```python
from build123d import *

# Parameters (mm, degrees)
F0_W     = 32
F0_H     = 32
F1_DEPTH = 1.6
F2_W     = 5.95
F2_H     = 3.7
F3_DEPTH = 4.75
F4_W     = 16.95
F4_H     = 16.95
F5_DEPTH = 7.75
F6_R     = 7.575
F7_DEPTH = 15.5
F8_R     = 1
F9_DEPTH = 7.75


# Not quite as in the source:
# - a pattern or mirror of a feature is missing from the dataset's text; its kind, count and spacing are read off the source's solid


with BuildPart() as f1:
    # F0 (on Front) → F1 (new body)
    with BuildSketch(Plane.XZ):
        Rectangle(F0_W, F0_H)
    extrude(amount=F1_DEPTH)

    # F2 (on face) → F3 (join)
    with BuildSketch(Plane.XZ.offset(1.6)):
        with Locations((-7.275, -14.15)):
            Rectangle(F2_W, F2_H)
    extrude(amount=F3_DEPTH)

    # F4 (on face) → F5 (join)
    with BuildSketch(Plane(origin=(0, 0, 0), x_dir=(-1, 0, 0), z_dir=(0, 1, 0))):
        Rectangle(F4_W, F4_H)
    extrude(amount=F5_DEPTH)

    # F6 (on face) → F7 (join)
    with BuildSketch(Plane(origin=(0, 7.75, 0), x_dir=(-1, 0, 0), z_dir=(0, 1, 0))):
        Circle(F6_R)
    extrude(amount=F7_DEPTH)

    # F8 (on face) → F9 (join)
    with BuildSketch(Plane(origin=(0, 0, 0), x_dir=(-1, 0, 0), z_dir=(0, 1, 0))):
        with BuildLine():
            Line((-8.475, 2.4), (-10, 2.4))
            ThreePointArc((-10, 2.4), (-12.4, 0), (-10, -2.4))
            Line((-10, -2.4), (-8.475, -2.4))
            Line((-8.475, -2.4), (-8.475, 2.4))
        make_face()
        with Locations((-10, 0)):
            Circle(F8_R, mode=Mode.SUBTRACT)
    f9 = extrude(amount=F9_DEPTH)

    # F9_copies: F9 across plane
    add(f9.mirror(Plane(origin=(0, 0, 0), x_dir=(0, 0, -1), z_dir=(-1, 0, 0))))


solid = f1.part
```
Read the model definition and answer for the solid it produces. Units are mm, in the model's axes. A direction names the side the tool comes from. Give positions to 0.01 mm unless a question says otherwise; leave off trailing zeros. Loops run counter-clockwise (first coordinate to the right, second up) from the corner with the lowest first, then second, coordinate; pieces in that order, holes last.
Item 1: The mould has two halves that part along Z. Classify faces 1 (the flat face through (-10, 0, 0)), 2 (the cylindrical face through (-10.8, 3.8, -0.6)), 3 (the flat face through (9, 4, 2.4)), 4 (the flat face through (9, 4, -2.4)): released by +Z, released by -Z, zero draft, split by the parting line, or undercut.
Item 2: Each of these flat-tipped pins is pushed along its axis until it touches: pin 1 Ø2.5 at (x, z) = (-10, 0) entering from -Y; pin 2 Ø0.6 at (x, z) = (-10, -0.5) entering from +Y; pin 3 Ø5 at (x, y) = (-9.5, 14.5) entering from -Z. Where does it stop, or does it pass through?
Item 3: For faces 5 (the flat face through (0, 7.75, 8)), 6 (the flat face through (-10.25, -4, -14)), 7 (the flat face through (0, 4, -8.475)), 8 (the cylindrical face through (-12.4, 3.82, 0.05)), determine the directions among +Z, -Z, +X, -X, +Y, -Y from which every point of the face is accessible in a straight line to the end or side of a thin tool.
Item 4: The part is cut by section C-C (x = 0). Write down the section's boundary in (y, z) (3 decimals), and give its area (3 significant figures).
Item 5: The part is cut by section A-A (y = 0.5). Write down the section's boundary in (x, z) (3 decimals).
Item 6: Find the intervals of material crossed by line 1 along Z through (x, y) = (-10, 6); line 2 along Y through (x, z) = (3, 12); line 3 along Y through (x, z) = (1, -7), in increasing order.
Item 7: The part is cut by section B-B (z = 0). Write down the section's boundary in (x, y) (3 decimals).
Item 8: The part is cut by section D-D (y = 16.5). Write down the section's boundary in (x, z) (3 decimals).
Taken from the geometry:
1. face 1: undercut
1. face 2: undercut
1. face 3: released by +Z
1. face 4: released by -Z
2. pin 1: stops at y = -1.6
2. pin 2: stops at y = 0
2. pin 3: stops at z = -2.89
3. face 5: +Y
3. face 6: +Z, -Z, -X, -Y
3. face 7: -Z, +X, -X, +Y
3. face 8: -X, +Y
4. outline: (-1.6, -16) - (0, -16) - (0, -8.475) - (7.75, -8.475) - (7.75, -7.575) - (23.25, -7.575) - (23.25, 7.575) - (7.75, 7.575) - (7.75, 8.475) - (0, 8.475) - (0, 16) - (-1.6, 16) - close
4. area: 417 mm2
5. outline: (-10, -2.4) - (-8.475, -2.4) - (-8.475, -8.475) - (8.475, -8.475) - (8.475, -2.4) - (10, -2.4) arc R2.4 ccw to (10, 2.4) - (8.475, 2.4) - (8.475, 8.475) - (-8.475, 8.475) - (-8.475, 2.4) - (-10, 2.4) arc R2.4 ccw to start; hole circle Ø2 at (-10, 0); hole circle Ø2 at (10, 0)
6. line 1: z = -2.4 to -1, 1 to 2.4
6. line 2: y = -1.6 to 0
6. line 3: y = -1.6 to 23.25
7. outline: (-16, -1.6) - (16, -1.6) - (16, 0) - (12.4, 0) - (12.4, 7.75) - (11, 7.75) - (11, 0) - (9, 0) - (9, 7.75) - (7.575, 7.75) - (7.575, 23.25) - (-7.575, 23.25) - (-7.575, 7.75) - (-9, 7.75) - (-9, 0) - (-11, 0) - (-11, 7.75) - (-12.4, 7.75) - (-12.4, 0) - (-16, 0) - close
8. outline: circle Ø15.15 at (0, 0)
